Model file for the job. Use its own axes, mm. A direction names the side the tool comes from. Coordinates: 2 decimals unless noted, no trailing zeros. Write each loop counter-clockwise with the first axis right and the second up, starting at its lowest first coordinate (ties: lowest second). Pieces come first, ordered by that corner, then holes.
Q1. Which spindle directions (+Z, -Z, +X, -X, +Y, -Y) get a long thin tool onto all of the face, cutting with end or side? Do faces 1 (the flat face through (7, -12, -36.754)), 2 (the flat face through (7, -12, 51.227)), 3 (the cylindrical face through (7.337, -23.496, -35.328)), 4 (the cylindrical face through (9.2, -23.5, 49.8)). Say none if no direction does.
Q2. Band-saw the part on B-B, the plane y = -8.75. Write the cut outline in (x, z).
Q3. Pin check, flat tips, straight feed: P1, Ø12, axis at x = -5, y = -15.5, coming from the +Z side; P2, Ø6, axis at x = -114, y = -12.5, coming from the +Z side; P3, Ø1.5, axis at y = -15, z = -21, coming from the -X side; P4, Ø12, axis at x = -85, z = 43.5, coming from the +Y side. Stop position of each tip, or through.
Q4. Band-saw the part on C-C, the plane y = -22.5. Write the cut outline in (x, z).
Q5. Band-saw the part on A-A, the plane x = 58. Write the cut outline in (y, z), plus the area to 3 significant figures.
Q6. Drill centre lines: probe 1 along Z at (x, y) = (45.5, -6.75); probe 2 along Z at (x, y) = (46, -20.5); probe 3 along X at (y, z) = (-17.75, 36). Where is each one in solid material? Low to high.
from build123d import *

# Parameters (mm, degrees)
F0_W     = 179.208383
F0_H     = 87.981586
F1_DEPTH = 25
F2_R     = 59.70905
F3_DEPTH = 25
F4_R     = 15
F5_R     = 5
F6_SIZE  = 5


with BuildPart() as f1:
    # F0 (on Front) → F1 (new body)
    with BuildSketch(Plane.XZ):
        with Locations((-14.650919, 7.236587)):
            Rectangle(F0_W, F0_H)
    extrude(amount=F1_DEPTH)

    # F2 (on face) → F3 (join, through all)
    with BuildSketch(Plane.XZ.offset(25)):
        with Locations((-104.25511, 7.236587)):
            Circle(F2_R)
    extrude(amount=-F3_DEPTH)

    # F4
    f4_edges = [f1.edges().sort_by_distance(p)[0] for p in [
        (-63.882089, -12.5, 51.22738),
        (-63.882089, -12.5, -36.754206),
    ]]
    fillet(f4_edges, radius=F4_R)

    # F5
    f5_edges = [f1.edges().sort_by_distance(p)[0] for p in [
        (8.270297, -25, 51.22738),
        (-63.277779, -25, 52.038271),
        (74.953273, -25, 7.236587),
        (-163.96416, -25, 7.236587),
        (8.270297, -25, -36.754206),
        (-63.277779, -25, -37.565098),
    ]]
    fillet(f5_edges, radius=F5_R)

    # F6
    f6_edges = [f1.edges().sort_by_distance(p)[0] for p in [
        (8.270297, 0, 51.22738),
        (-63.277779, 0, 52.038271),
        (74.953273, 0, 7.236587),
        (-163.96416, 0, 7.236587),
        (8.270297, 0, -36.754206),
        (-63.277779, 0, -37.565098),
    ]]
    chamfer(f6_edges, length=F6_SIZE)


solid = f1.part
Answer sheet:
1. face 1: -Z, +X, +Y, -Y
1. face 2: +Z, +X, +Y, -Y
1. face 3: -Z, +X, -Y
1. face 4: +Z, +X, -Y
2. outline: (-67.62, -39.91) arc R15 cw to (-58.41, -36.75) - (74.95, -36.75) - (74.95, 51.23) - (-58.41, 51.23) arc R15 cw to (-67.62, 54.38) arc R59.71 ccw (long way) to start
3. P1: stops at z = 51.23
3. P2: stops at z = 66.56
3. P3: stops at x = -157.26
3. P4: stops at y = 0
4. outline: (-68.03, -39.38) arc R15.67 cw to (-58.41, -36.08) - (74.28, -36.08) - (74.28, 50.56) - (-58.41, 50.56) arc R15.67 cw to (-68.03, 53.85) arc R59.04 ccw (long way) to start
5. outline: (-25, -31.75) arc R5 ccw to (-20, -36.75) - (-5, -36.75) - (0, -31.75) - (0, 46.23) - (-5, 51.23) - (-20, 51.23) arc R5 ccw to (-25, 46.23) - close
5. area: 2,160 mm2
6. probe 1: z = -36.75 to 51.23
6. probe 2: z = -36.73 to 51.2
6. probe 3: x = -156.58 to 74.95
